Drawing for the job (mm, zero at the part's lowest x, y, z). Round coordinates to 2 decimals unless told otherwise and drop trailing zeros. Write each loop counter-clockwise with the first axis right and the second up, starting at its lowest first coordinate (ties: lowest second). Pieces come first, ordered by that corner, then holes. Notation, with made-up numbers: M 5.5,69 L 62.5,69 A19 cw 62.5,94 Z; hole C 85.25,50.25 d10. An arc over 180 degrees is marked long. Use a Markdown table: item, result. Add a question column.
1) Wall check: probe 1 along X at (y, z) = (0.95, 49); probe 2 along X at (y, z) = (0.65, 21); probe 3 along Z at (x, y) = (30, 0.3) (1 decimal). Give the ranges that are in metal, low to high.
2) Slice it at D-D on z = 30.5. Write the cut outline in (x, y) (1 decimal).
3) Slice it at C-C on x = 16. Write the cut outline in (y, z).
4) Slice it at B-B on z = 59. Write the cut outline in (x, y), plus the area to 3 significant figures.
5) Slice it at A-A on x = 21. Write the cut outline in (y, z).
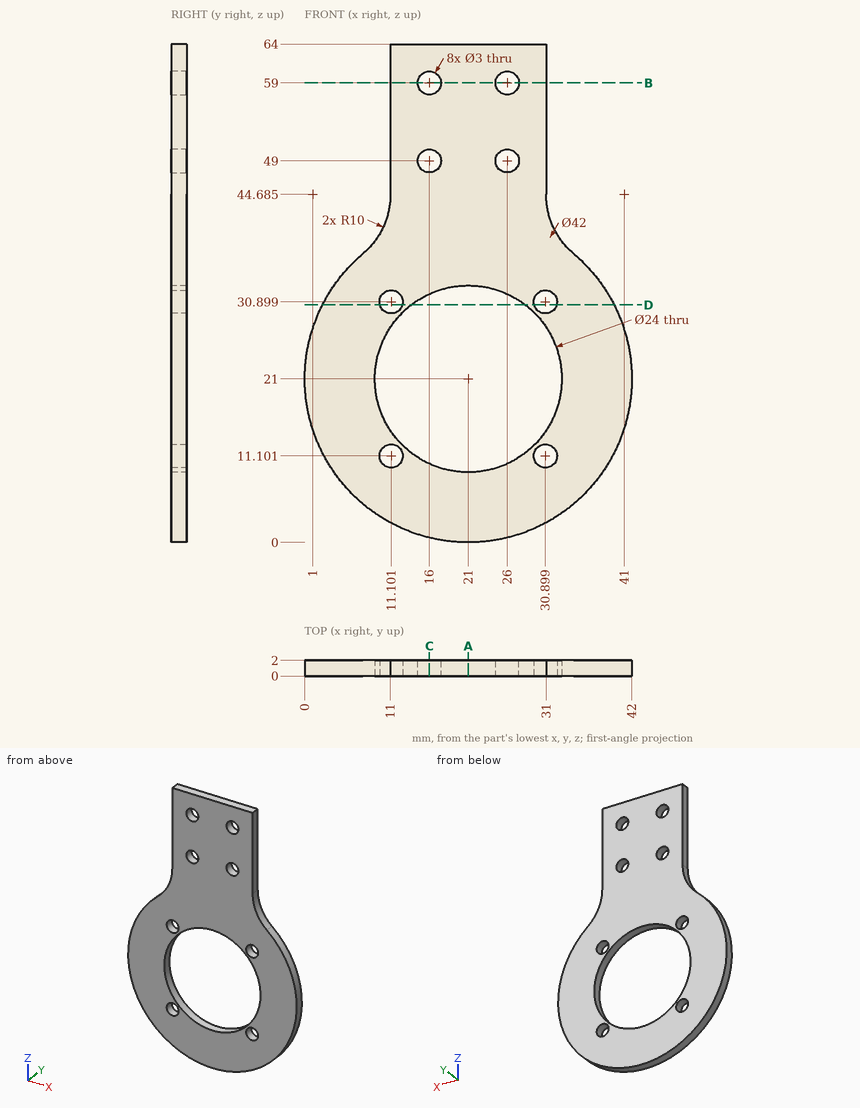
Entries:
| question | item | result |
|---|---|---|
| 1 | probe 1 | x = 11 to 14.5, 17.5 to 24.5, 27.5 to 31 |
| 1 | probe 2 | x = 0 to 9, 33 to 42 |
| 1 | probe 3 | z = 2 to 9.9, 12.3 to 13.1, 28.9 to 29.7, 32.1 to 64 |
| 2 | outline | M 2.3,0 L 9.7,0 L 9.7,2 L 2.3,2 Z; M 12.5,0 L 13.7,0 L 13.7,2 L 12.5,2 Z; M 28.3,0 L 29.5,0 L 29.5,2 L 28.3,2 Z; M 32.3,0 L 39.7,0 L 39.7,2 L 32.3,2 Z |
| 3 | outline | M 0,0.6 L 2,0.6 L 2,10.09 L 0,10.09 Z; M 0,31.91 L 2,31.91 L 2,47.5 L 0,47.5 Z; M 0,50.5 L 2,50.5 L 2,57.5 L 0,57.5 Z; M 0,60.5 L 2,60.5 L 2,64 L 0,64 Z |
| 4 | outline | M 11,0 L 14.5,0 L 14.5,2 L 11,2 Z; M 17.5,0 L 24.5,0 L 24.5,2 L 17.5,2 Z; M 27.5,0 L 31,0 L 31,2 L 27.5,2 Z |
| 4 | area | 28.0 mm^2 |
| 5 | outline | M 0,0 L 2,0 L 2,9 L 0,9 Z; M 0,33 L 2,33 L 2,64 L 0,64 Z |
